Part model, mm, in its own coordinate system. A direction names the side the tool comes from. Give positions to 0.01 mm unless a question says otherwise; leave off trailing zeros. Write each loop counter-clockwise with the first axis right and the second up, starting at its lowest first coordinate (ties: lowest second). Pieces come first, ordered by that corner, then holes.
from build123d import *

# Parameters (mm, degrees)
SKETCH_1_W          = 7.5
SKETCH_1_H          = 3
EXTRUDE_1_DEPTH     = 4.5
SKETCH_2_W          = 1.2
SKETCH_2_H          = 2.5
EXTRUDE_2_DEPTH     = 1.6
CUT_EXTRUDE_1_DEPTH = 10.39853712


with BuildPart() as part:
    # 草图1 → 凸台-拉伸1 (new body)
    with BuildSketch(Plane(origin=(0, 0, 0), x_dir=(1, 0, 0), z_dir=(0, 1, 0))):
        with Locations((-3.75, 1.5)):
            Rectangle(SKETCH_1_W, SKETCH_1_H)
    extrude(amount=EXTRUDE_1_DEPTH)

    # 草图2 → 凸台-拉伸2 (add)
    with BuildSketch(Plane(origin=(0, 0, -3), x_dir=(-1, 0, 0), z_dir=(0, 0, -1))):
        with Locations((1.25, 2.45)):
            Rectangle(SKETCH_2_W, SKETCH_2_H)
        with Locations((3.75, 2.45)):
            Rectangle(SKETCH_2_W, SKETCH_2_H)
        with Locations((6.25, 2.45)):
            Rectangle(SKETCH_2_W, SKETCH_2_H)
    extrude(amount=EXTRUDE_2_DEPTH)

    # 草图3 → 切除-拉伸1 (cut, through all)
    with BuildSketch(Plane(origin=(-0.65, 0, 0), x_dir=(0, 0, -1), z_dir=(1, 0, 0))):
        with BuildLine():
            add(Edge.make_bspline(
                [(4.6, 2.45), (4.6, 3.075), (3, 3.7)],
                knots=[0.5, 0.5, 0.5, 1, 1, 1], degree=2))
            Line((4.6, 2.45), (4.6, 3.7))
            Line((4.6, 3.7), (3, 3.7))
        make_face()
        with BuildLine():
            add(Edge.make_bspline(
                [(3, 1.2), (4.6, 1.825), (4.6, 2.45)],
                knots=[0, 0, 0, 0.5, 0.5, 0.5], degree=2))
            Line((3, 1.2), (4.6, 1.2))
            Line((4.6, 1.2), (4.6, 2.45))
        make_face()
    extrude(amount=-CUT_EXTRUDE_1_DEPTH, mode=Mode.SUBTRACT)


solid = part.part
1) Saw through at B-B (z = -3.3). State how many separate pieces and enclosed holes the cut face has, and give its area (3 significant figures).
Check result:
separate pieces: 3
enclosed holes: 0
area: 8.11 mm2
2) Mould opens along X. For faces 1 (the flat face through (-6.85, 2, -4)), 2 (the flat face through (-4, 0, -2)), 3 (the flat face through (-3.15, 2, -4)) say: +X half, -X half, draft (parallel to the pull), parting line (faces both ways), or undercut.
Check result:
face 1: -X half
face 2: draft
face 3: undercut
3) Saw through at A-A (y = 1.1). Write the cut outline in (x, z), and give its area (3 significant figures).
Check result:
outline: (-7.5, -3) - (0, -3) - (0, 0) - (-7.5, 0) - close
area: 22.5 mm2
4) Flat gauge pins, fed straight in: P1, Ø0.8, axis at y = 2, z = -3.5, coming from the +X side; P2, Ø0.8, axis at y = 2, z = -4, coming from the -X side. Where does each tip first touch, or does it go through?
Check result:
P1: stops at x = -0.65
P2: stops at x = -6.85
5) Drill centre lines: L1, parallel to Z at x = -3.75, y = 0.95; L2, parallel to Z at x = -5.75, y = 1.7. Where is each one in solid material? Low to high.
Check result:
L1: z = -3 to 0
L2: z = -4.02 to 0
6) Saw through at C-C (x = -5.5). Write the cut outline in (y, z).
Check result:
outline: (0, -3) - (4.5, -3) - (4.5, 0) - (0, 0) - close
7) 3-axis set-ups, long thin cutter, end or side, ignore diameter. For faces 4 (the flat face through (-4.35, 2, -4)), 5 (the flat face through (-7.5, 2, -1)), 6 (the flat face through (-0.65, 2, -4)): which of +Z, -Z, +X, -X, +Y, -Y reach the whole face in a straight line?
Check result:
face 4: -Z, +Y, -Y
face 5: +Z, -Z, -X, +Y, -Y
face 6: -Z, +X, +Y, -Y
